```python
from build123d import *

# Parameters (mm, degrees)
F1_DEPTH = 45.025
F3_DEPTH = 35


with BuildPart() as f1:
    # F0 (on Front) → F1 (new body)
    with BuildSketch(Plane.XZ):
        Polygon((18.4, 0), (0, 0), (0, -14), (16.314836, -37.3), (17.339836, -37.3), (17.339836, -38.763852), (17.715251, -39.3), (17.339836, -39.836148), (17.339836, -41.3), (16.314836, -41.3), (0, -64.6), (0, -78.6), (21.8, -78.6), (31.5, -71.807987), (31.5, -70.782987), (32.963852, -70.782987), (33.5, -70.407572), (34.036148, -70.782987), (35.5, -70.782987), (35.5, -71.807987), (45.2, -78.6), (67, -78.6), (67, -58.8), (54.746368, -41.3), (53.721368, -41.3), (53.721368, -39.836148), (53.345953, -39.3), (53.721368, -38.763852), (53.721368, -37.3), (54.746368, -37.3), (67, -19.8), (67, 0), (48.6, 0), (35.5, -9.172719), (35.5, -10.197719), (34.036148, -10.197719), (33.5, -10.573134), (32.963852, -10.197719), (31.5, -10.197719), (31.5, -9.172719), align=None)
        Polygon((53.721368, -39.836148), (53.721368, -38.763852), (53.345953, -39.3), align=None)
        Polygon((17.715251, -39.3), (17.339836, -38.763852), (17.339836, -39.836148), align=None)
        Polygon((34.036148, -10.197719), (32.963852, -10.197719), (33.5, -10.573134), align=None)
        Polygon((33.5, -70.407572), (32.963852, -70.782987), (34.036148, -70.782987), align=None)
    extrude(amount=F1_DEPTH)

    # F2 (on face) → F3 (cut)
    with BuildSketch(Plane.XZ.offset(45.025)):
        Polygon((28.632118, -13.268479), (16.823506, -5), (5, -5), (5, -12.423506), (20.410596, -34.432118), (23.819123, -39.299999), (20.410595, -44.167881), (4.999998, -66.176493), (4.999998, -73.600002), (20.223507, -73.600002), (28.632119, -67.712228), (33.500001, -64.3037), (38.367882, -67.712227), (46.776494, -73.6), (62, -73.6), (62, -60.376494), (50.650608, -44.167882), (47.24208, -39.3), (50.650608, -34.432118), (62, -18.223506), (62, -5), (50.176494, -5), (38.367882, -13.268479), (33.5, -16.677007), align=None)
    extrude(amount=-F3_DEPTH, mode=Mode.SUBTRACT)

    # F4: F1 across face


with BuildPart() as f1_1:
    add(f1.part)
    add(f1.part.mirror(Plane(origin=(34.584807, 0, -39.813495), x_dir=(1, 0, 0), z_dir=(0, 1, 0))))


solid = f1_1.part
```
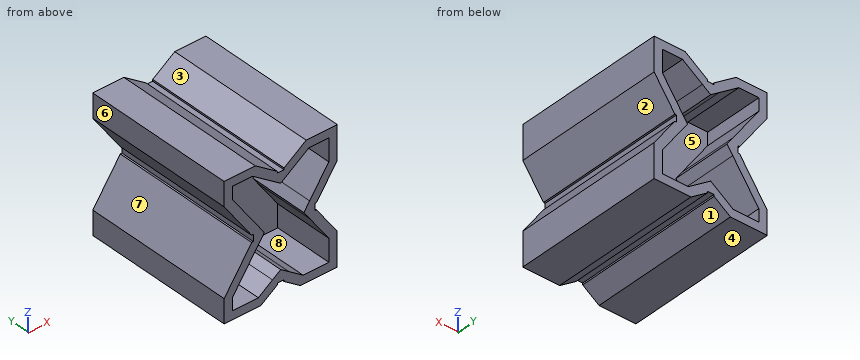
Part model, mm, in its own coordinate system. Face numbers are marked on the shaded views. A direction names the side the tool comes from. Round coordinates to 2 decimals unless told otherwise and drop trailing zeros. Write each loop counter-clockwise with the first axis right and the second up, starting at its lowest first coordinate (ties: lowest second). Pieces come first, ordered by that corner, then holes.
Item 1: Two-plate mould, pull along Z, no slides. Class the marked faces 1, 2 and 3: +Z half, -Z half, draft (parallel to the pull), parting line (faces both ways), or undercut.
Results:
face 1: -Z half
face 2: undercut
face 3: +Z half
Item 2: Which spindle directions (+Z, -Z, +X, -X, +Y, -Y) get a long thin tool onto all of the face, cutting with end or side? Do the marked faces 4, 5, 6, 7 and 8. Say none if no direction does.
Results:
face 4: -Z, +X, -X, +Y, -Y
face 5: +Y
face 6: +Z, -Z, -X, +Y, -Y
face 7: -X, +Y, -Y
face 8: -Y
Item 3: Probe L1, parallel to X at y = -0.5, z = -71; L2, parallel to X at y = -17.5, z = -64.5; L3, parallel to X at y = -29, z = -9. List the from-to ranges inside material, lowest first.
Results:
L1: x = 0 to 31.5, 35.5 to 67
L2: x = 0.07 to 6.17, 33.22 to 33.78, 62 to 67
L3: x = 0 to 5, 22.54 to 31.25, 35.75 to 44.46, 62 to 67
Item 4: Cut at A-A, the plane x = 10. Give the cut face in (y, z) (3 decimals).
Results:
outline: (-45.025, -78.6) - (45.025, -78.6) - (45.025, -73.6) - (10.025, -73.6) - (10.025, -59.036) - (45.025, -59.036) - (45.025, -50.319) - (-45.025, -50.319) - (-45.025, -59.036) - (-10.025, -59.036) - (-10.025, -73.6) - (-45.025, -73.6) - close; (-45.025, -28.281) - (45.025, -28.281) - (45.025, -19.564) - (10.025, -19.564) - (10.025, -5) - (45.025, -5) - (45.025, 0) - (-45.025, 0) - (-45.025, -5) - (-10.025, -5) - (-10.025, -19.564) - (-45.025, -19.564) - close
Item 5: Cut at B-B, the plane y = 5. Give the cut face in (x, z).
Results:
outline: (0, -78.6) - (21.8, -78.6) - (31.5, -71.81) - (31.5, -70.78) - (35.5, -70.78) - (35.5, -71.81) - (45.2, -78.6) - (67, -78.6) - (67, -58.8) - (54.75, -41.3) - (53.72, -41.3) - (53.72, -37.3) - (54.75, -37.3) - (67, -19.8) - (67, 0) - (48.6, 0) - (35.5, -9.17) - (35.5, -10.2) - (31.5, -10.2) - (31.5, -9.17) - (18.4, 0) - (0, 0) - (0, -14) - (16.31, -37.3) - (17.34, -37.3) - (17.34, -41.3) - (16.31, -41.3) - (0, -64.6) - close
Item 6: Cut at D-D, the plane x = 42.5. Give the cut face in (y, z) (3 decimals).
Results:
outline: (-45.025, -76.709) - (45.025, -76.709) - (45.025, -70.606) - (10.025, -70.606) - (10.025, -10.375) - (45.025, -10.375) - (45.025, -4.271) - (-45.025, -4.271) - (-45.025, -10.375) - (-10.025, -10.375) - (-10.025, -70.606) - (-45.025, -70.606) - close
Item 7: Drop flat-ended pins along their axis: pin 1 Ø2 at (x, z) = (28.5, -46.5) entering from +Y (3 decimals); pin 2 Ø1 at (y, z) = (21.5, -41.5) entering from +X; pin 3 Ø3 at (x, y) = (32.5, -15) entering from +Z. Give the stop position or say it passes through.
Results:
pin 1: stops at y = 10.025
pin 2: stops at x = 55.24
pin 3: stops at z = -8.82
Item 8: Cut at C-C, the plane z = -25. Give the cut face in (x, y) (3 decimals).
Results:
outline: (7.702, -45.025) - (13.806, -45.025) - (13.806, -10.025) - (57.255, -10.025) - (57.255, -45.025) - (63.359, -45.025) - (63.359, 45.025) - (57.255, 45.025) - (57.255, 10.025) - (13.806, 10.025) - (13.806, 45.025) - (7.702, 45.025) - close
